```python
from build123d import *

# Parameters (mm, degrees)
SKETCH1_W           = 100
SKETCH1_H           = 210
BOSS_EXTRUDE1_DEPTH = 10
SKETCH2_W           = 30
SKETCH2_H           = 185
CUT_EXTRUDE2_DEPTH  = 8
BOSS_EXTRUDE3_DEPTH = 30
SKETCH4_W           = 200
SKETCH4_H           = 7.5
CUT_EXTRUDE3_DEPTH  = 10
SKETCH5_W           = 200
SKETCH5_H           = 7.5
CUT_EXTRUDE4_DEPTH  = 10
SKETCH6_W           = 15
SKETCH6_H           = 15
CUT_EXTRUDE5_DEPTH  = 2


with BuildPart() as part:
    # Sketch1 → Boss-Extrude1 (new body)
    with BuildSketch(Plane(origin=(0, 0, 0), x_dir=(1, 0, 0), z_dir=(0, 1, 0))):
        with Locations((50, -105)):
            Rectangle(SKETCH1_W, SKETCH1_H)
    extrude(amount=BOSS_EXTRUDE1_DEPTH)

    # Sketch2 → Cut-Extrude2 (cut)
    with BuildSketch(Plane(origin=(0, 10, 0), x_dir=(1, 0, 0), z_dir=(0, 1, 0))):
        with Locations((50, -117.5)):
            Rectangle(SKETCH2_W, SKETCH2_H)
    extrude(amount=-CUT_EXTRUDE2_DEPTH, mode=Mode.SUBTRACT)

    # Sketch3 → Boss-Extrude3 (add)
    with BuildSketch(Plane.ZY.offset(-65)):
        Polygon((25, 2), (65, 2), (25, 10), align=None)
    extrude(amount=BOSS_EXTRUDE3_DEPTH)

    # Sketch4 → Cut-Extrude3 (cut)
    with BuildSketch(Plane(origin=(100, 0, 0), x_dir=(0, 0, -1), z_dir=(1, 0, 0))):
        with Locations((-105, 3.75)):
            Rectangle(SKETCH4_W, SKETCH4_H)
    extrude(amount=-CUT_EXTRUDE3_DEPTH, mode=Mode.SUBTRACT)

    # Sketch5 → Cut-Extrude4 (cut)
    with BuildSketch(Plane.ZY):
        with Locations((105, 3.75)):
            Rectangle(SKETCH5_W, SKETCH5_H)
    extrude(amount=-CUT_EXTRUDE4_DEPTH, mode=Mode.SUBTRACT)

    # Sketch6 → Cut-Extrude5 (cut)
    with BuildSketch(Plane(origin=(0, 10, 0), x_dir=(1, 0, 0), z_dir=(0, 1, 0))):
        with Locations((25.5, -32.5)):
            Rectangle(SKETCH6_W, SKETCH6_H)
        with Locations((74.5, -32.5)):
            Rectangle(SKETCH6_W, SKETCH6_H)
    extrude(amount=-CUT_EXTRUDE5_DEPTH, mode=Mode.SUBTRACT)


solid = part.part
```
The listing builds one solid part. Answer for the finished solid, in the listing's coordinates (mm). A direction names the side the tool comes from. Give positions to 0.01 mm unless a question says otherwise; leave off trailing zeros. Write each loop counter-clockwise with the first axis right and the second up, starting at its lowest first coordinate (ties: lowest second). Pieces come first, ordered by that corner, then holes. Notation, with made-up numbers: (76.25, 56.25) -> (121.25, 56.25) arc R19 cw to (121.25, 89.25) -> close; hole circle Ø7 at (43, 28). An arc over 180 degrees is marked (long way). Write item = value, one per line. Start each with the question number.
1) Each of these flat-tipped pins is pushed along its axis until it touches: pin 1 (9 mm diameter, centred on x = 51, z = 141, fed in from +Y); pin 2 (2 mm diameter, centred on y = 4.5, z = 60.5, fed in from -X); pin 3 (4 mm diameter, centred on y = 2, z = 67, fed in from +X). Where does it stop, or does it pass through?
2) Straight lines are drawn through the part: line 1 along X through (y, z) = (6.5, 119); line 2 along X through (y, z) = (8.5, 160); line 3 along Y through (x, z) = (71.5, 31). For each, find the intervals that lie inside material, in ascending order.
3) Which of the six approach directions +Z, -Z, +X, -X, +Y, -Y give full straight-line access (tool end or side, diameter ignored) to faces 4 (the face through (74, 8, 32)), 5 (the face through (65, 6, 119)), 6 (the face through (5, 4, 5)), 7 (the face through (90, 4, 106))?
4) The part is cut by section A-A, the plane z = 122.5. Determine the outline of the cut face in (x, y).
5) The part is cut by section C-C, the plane z = 51. Determine the outline of the cut face in (x, y), and give its area (3 significant figures).
6) The part is cut by section B-B, the plane x = 49.5. Determine the outline of the cut face in (y, z).
7) Determine the mould class of faces 1 (the face through (49, 5, 0)), 2 (the face through (49, 0, 104)), 3 (the face through (95, 4, 205)) for opening direction Z: +Z half, -Z half, draft (parallel to the pull), parting line (faces both ways), or undercut.
Solutions:
q1.pin_1 = 2
q1.pin_2 = 10
q1.pin_3 = 90
q2.line_1 = 10 to 35, 65 to 90
q2.line_2 = 0 to 35, 65 to 100
q2.line_3 = 0 to 8
q3.face_4 = +Y
q3.face_5 = +Z, +Y
q3.face_6 = -X, -Y
q3.face_7 = +X, -Y
q4.outline = (0, 7.5) -> (10, 7.5) -> (10, 0) -> (90, 0) -> (90, 7.5) -> (100, 7.5) -> (100, 10) -> (65, 10) -> (65, 2) -> (35, 2) -> (35, 10) -> (0, 10) -> close
q5.outline = (0, 7.5) -> (10, 7.5) -> (10, 0) -> (90, 0) -> (90, 7.5) -> (100, 7.5) -> (100, 10) -> (65, 10) -> (65, 4.8) -> (35, 4.8) -> (35, 10) -> (0, 10) -> close
q5.area = 694 mm²
q6.outline = (0, 0) -> (10, 0) -> (10, 25) -> (2, 65) -> (2, 210) -> (0, 210) -> close
q7.face_1 = -Z half
q7.face_2 = draft
q7.face_3 = undercut
